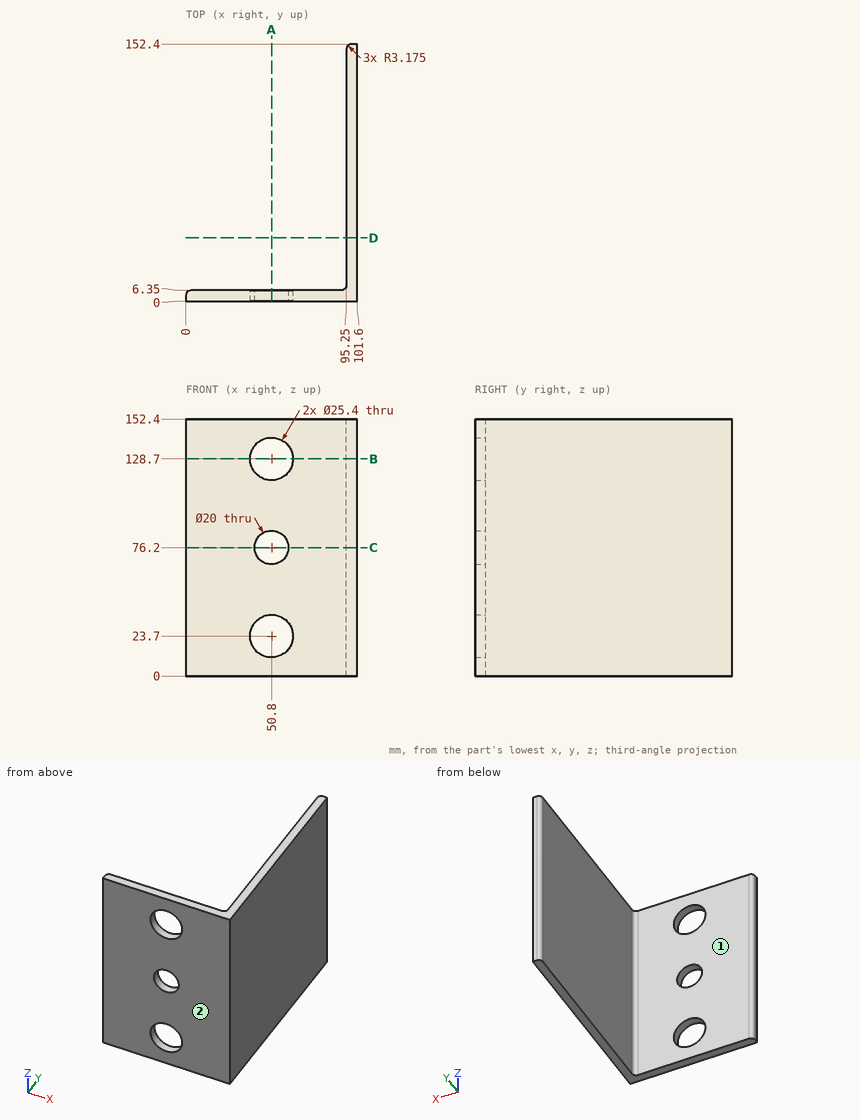
Geometry check sheet. Reference: drawing and pictorial views, mm from the part's lowest x, y, z. A direction names the side the tool comes from. Give positions to 0.01 mm unless a question says otherwise; leave off trailing zeros. Write each loop counter-clockwise with the first axis right and the second up, starting at its lowest first coordinate (ties: lowest second). Pieces come first, ordered by that corner, then holes.
Item 1: Cross-section at B-B (z = 128.7). Enter the section's corners in (x, y) (3 decimals), and give its area (3 significant figures).
Item 2: Gauge pin test, flat ends, axial feed: pin 1 (3 mm diameter, centred on x = 13.5, z = 136, fed in from +Y); pin 2 (3 mm diameter, centred on y = 31.5, z = 74.5, fed in from -X). Record the tip position at first contact, or that the pin passes through.
Item 3: Scan lines: L1, parallel to Z at x = 50, y = 1; L2, parallel to X at y = 2.75, z = 128.7; L3, parallel to X at y = 2.25, z = 76.2. Record each from-to range of solid material in increasing order.
Item 4: Cross-section at C-C (z = 76.2). Enter the section's corners in (x, y) (3 decimals), and give its area (3 significant figures).
Item 5: Cross-section at A-A (x = 50.8). Enter the section's corners in (y, z), and give its area (3 significant figures).
Item 6: Access from +Z, -Z, +X, -X, +Y, -Y to the whole of each face (thin tool, end or side, straight path). Record for the marked faces 1 and 2.
Item 7: Cross-section at D-D (y = 37.5). Enter the section's corners in (x, z), and give its area (3 significant figures).
Report:
1. outline: (0, 0) - (38.1, 0) - (38.1, 6.35) - (3.175, 6.35) arc R3.175 ccw to (0, 3.175) - close; (63.5, 0) - (101.6, 0) - (101.6, 152.4) - (98.425, 152.4) arc R3.175 ccw to (95.25, 149.225) - (95.25, 9.525) arc R3.175 cw to (92.075, 6.35) - (63.5, 6.35) - close
1. area: 1,410 mm2
2. pin 1: stops at y = 6.35
2. pin 2: stops at x = 95.25
3. L1: z = 0 to 11.03, 36.37 to 66.23, 86.17 to 116.03, 141.37 to 152.4
3. L2: x = 0 to 38.1, 63.5 to 101.6
3. L3: x = 0 to 40.8, 60.8 to 101.6
4. outline: (0, 0) - (40.8, 0) - (40.8, 6.35) - (3.175, 6.35) arc R3.175 ccw to (0, 3.175) - close; (60.8, 0) - (101.6, 0) - (101.6, 152.4) - (98.425, 152.4) arc R3.175 ccw to (95.25, 149.225) - (95.25, 9.525) arc R3.175 cw to (92.075, 6.35) - (60.8, 6.35) - close
4. area: 1,440 mm2
5. outline: (0, 0) - (6.35, 0) - (6.35, 11) - (0, 11) - close; (0, 36.4) - (6.35, 36.4) - (6.35, 66.2) - (0, 66.2) - close; (0, 86.2) - (6.35, 86.2) - (6.35, 116) - (0, 116) - close; (0, 141.4) - (6.35, 141.4) - (6.35, 152.4) - (0, 152.4) - close
5. area: 518 mm2
6. face 1: +Z, -Z, -X, +Y
6. face 2: +Z, -Z, +X, -X, -Y
7. outline: (95.25, 0) - (101.6, 0) - (101.6, 152.4) - (95.25, 152.4) - close
7. area: 968 mm2
